Work out the finished part from the listing and answer in its coordinate system (mm). A direction names the side the tool comes from. Give positions to 0.01 mm unless a question says otherwise; leave off trailing zeros. Loops run counter-clockwise (first coordinate to the right, second up) from the corner with the lowest first, then second, coordinate; pieces in that order, holes last. Notation, with made-up numbers: (31.25, 38) - (61.25, 38) arc R24 cw to (61.25, 55) - close; hole circle Ø2 at (-24.75, 44.5). An arc over 180 degrees is marked (long way). One line per item, written item: value.
from build123d import *

# Parameters (mm, degrees)
SKETCH_1_W           = 35.5
SKETCH_1_H           = 24
EXTRUDE_1_DEPTH      = 7
SKETCH_2_W           = 33.2
SKETCH_2_H           = 22.1
CUT_EXTRUDE_1_DEPTH  = 6
CUT_EXTRUDE_2_DEPTH  = 2
EXTRUDE_2_DEPTH      = 6
SKETCH_7_W           = 5
SKETCH_7_H           = 2
EXTRUDE_3_DEPTH      = 5
CUT_EXTRUDE_4_DEPTH  = 2
SKETCH_12_W          = 5.5
SKETCH_12_H          = 2
CUT_EXTRUDE_6_DEPTH  = 6
SKETCH_19_W          = 8
SKETCH_19_H          = 10
USB_DEPTH            = 1.5
SKETCH_25_W          = 0.5
SKETCH_25_H          = 18.1
CUT_EXTRUDE_12_DEPTH = 6
SKETCH_28_W          = 5.5
SKETCH_28_H          = 1.9
CUT_EXTRUDE_13_DEPTH = 6
SKETCH_29_W          = 6
SKETCH_29_H          = 2
CUT_EXTRUDE_14_DEPTH = 5
SKETCH_34_W          = 7
SKETCH_34_H          = 10
EXTRUDE_10_DEPTH     = 3.3
SKETCH_35_W          = 0.5
SKETCH_35_H          = 10
CUT_EXTRUDE_15_DEPTH = 3
SKETCH_37_W          = 4.5
SKETCH_37_H          = 2
EXTRUDE_12_DEPTH     = 5.5
SKETCH_38_W          = 1.5
SKETCH_38_H          = 2.5
CUT_EXTRUDE_16_DEPTH = 2
SKETCH_39_W          = 4.5
SKETCH_39_H          = 1
CUT_EXTRUDE_17_DEPTH = 5.5
SKETCH_40_W          = 4.5
SKETCH_40_H          = 3
EXTRUDE_13_DEPTH     = 1.5
FILLET_2_R           = 1
SKETCH_41_W          = 4.5
SKETCH_41_H          = 2
EXTRUDE_14_DEPTH     = 5.5
SKETCH_42_W          = 1.5
SKETCH_42_H          = 2.5
CUT_EXTRUDE_18_DEPTH = 2
SKETCH_43_W          = 4.5
SKETCH_43_H          = 1
CUT_EXTRUDE_19_DEPTH = 5.5
SKETCH_44_W          = 4.5
SKETCH_44_H          = 3
EXTRUDE_15_DEPTH     = 1.5
FILLET_3_R           = 1
EXTRUDE_16_DEPTH     = 2
SKETCH_50_W          = 5.5
SKETCH_50_H          = 2
CUT_EXTRUDE_20_DEPTH = 2
SKETCH_51_W          = 5.5
SKETCH_51_H          = 2
CUT_EXTRUDE_21_DEPTH = 2
SKETCH_54_W          = 2
SKETCH_54_H          = 0.95
EXTRUDE_19_DEPTH     = 2
SKETCH_55_W          = 2
SKETCH_55_H          = 1
EXTRUDE_20_DEPTH     = 15.5
SKETCH_56_W          = 2
SKETCH_56_H          = 1
EXTRUDE_21_DEPTH     = 2
SKETCH_57_W          = 2
SKETCH_57_H          = 1
EXTRUDE_22_DEPTH     = 7.5
SKETCH_58_W          = 1.5
SKETCH_58_H          = 1.9
SKETCH_58_H_2        = 2
EXTRUDE_24_DEPTH     = 2
SKETCH_59_W          = 6
SKETCH_59_H          = 1
EXTRUDE_25_DEPTH     = 1
CUT_EXTRUDE_22_DEPTH = 0.3
CUT_EXTRUDE_23_DEPTH = 0.3


with BuildPart() as part:
    # Sketch 1 → Extrude 1 (new body)
    with BuildSketch(Plane.XY):
        Rectangle(SKETCH_1_W, SKETCH_1_H)
    extrude(amount=EXTRUDE_1_DEPTH)

    # Sketch 2 → Cut-Extrude 1 (cut)
    with BuildSketch(Plane.XY.offset(7)):
        with Locations((0.25, 0.05)):
            Rectangle(SKETCH_2_W, SKETCH_2_H)
    extrude(amount=-CUT_EXTRUDE_1_DEPTH, mode=Mode.SUBTRACT)

    # Sketch 3 → Cut-Extrude 2 (cut)
    with BuildSketch(Plane.ZY.offset(17.75)):
        with BuildLine():
            Line((6, 7.45), (6, 1.95))
            ThreePointArc((6, 1.95), (4.25, 0.2), (2.5, 1.95))
            Line((2.5, 1.95), (2.5, 7.45))
            ThreePointArc((2.5, 7.45), (4.25, 9.2), (6, 7.45))
        make_face()
    extrude(amount=-CUT_EXTRUDE_2_DEPTH, mode=Mode.SUBTRACT)

    # Sketch 6 → Extrude 2 (add)
    with BuildSketch(Plane.XY.offset(1)):
        Polygon((-16.35, 10.1), (15.85, 10.1), (15.85, -10), (-16.35, -10), (-16.35, -11), (16.85, -11), (16.85, 11.1), (-16.35, 11.1), align=None)
    extrude(amount=EXTRUDE_2_DEPTH)

    # Sketch 7 → Extrude 3 (add)
    with BuildSketch(Plane.XY.offset(1)):
        with Locations((13.35, 9.1)):
            Rectangle(SKETCH_7_W, SKETCH_7_H)
    extrude(amount=EXTRUDE_3_DEPTH)

    # Sketch 10 → Cut-Extrude 4 (cut)
    with BuildSketch(Plane.ZY.offset(-15.85)):
        with BuildLine():
            Line((1.5, -6.45), (1.5, 4.55))
            ThreePointArc((1.5, 4.55), (3.75, 6.8), (6, 4.55))
            Line((6, 4.55), (6, -6.45))
            ThreePointArc((6, -6.45), (3.75, -8.7), (1.5, -6.45))
        make_face()
    extrude(amount=-CUT_EXTRUDE_4_DEPTH, mode=Mode.SUBTRACT)

    # Sketch 12 → Cut-Extrude 6 (cut)
    with BuildSketch(Plane.XY.offset(7)):
        with Locations((-1.6, -11)):
            Rectangle(SKETCH_12_W, SKETCH_12_H)
    extrude(amount=-CUT_EXTRUDE_6_DEPTH, mode=Mode.SUBTRACT)

    # Sketch 19 → USB (add)
    with BuildSketch(Plane.XY.offset(1)):
        with Locations((-12.25, 5.1)):
            Rectangle(SKETCH_19_W, SKETCH_19_H)
    extrude(amount=USB_DEPTH)

    # Sketch 25 → Cut-Extrude 12 (cut)
    with BuildSketch(Plane.XY.offset(7)):
        with Locations((16.1, -0.95)):
            Rectangle(SKETCH_25_W, SKETCH_25_H)
    extrude(amount=-CUT_EXTRUDE_12_DEPTH, mode=Mode.SUBTRACT)

    # Sketch 28 → Cut-Extrude 13 (cut)
    with BuildSketch(Plane.XY.offset(7)):
        with Locations((-5.1, 11.05)):
            Rectangle(SKETCH_28_W, SKETCH_28_H)
    extrude(amount=-CUT_EXTRUDE_13_DEPTH, mode=Mode.SUBTRACT)

    # Sketch 29 → Cut-Extrude 14 (cut)
    with BuildSketch(Plane.XY.offset(7)):
        with Locations((2.65, 11)):
            Rectangle(SKETCH_29_W, SKETCH_29_H)
    extrude(amount=-CUT_EXTRUDE_14_DEPTH, mode=Mode.SUBTRACT)

    # Sketch 34 → Extrude 10 (add)
    with BuildSketch(Plane.XY.offset(1)):
        with Locations((-12.75, -5)):
            Rectangle(SKETCH_34_W, SKETCH_34_H)
    extrude(amount=EXTRUDE_10_DEPTH)

    # Sketch 35 → Cut-Extrude 15 (cut)
    with BuildSketch(Plane.XY.offset(7)):
        with Locations((-16.5, 5.1)):
            Rectangle(SKETCH_35_W, SKETCH_35_H)
    extrude(amount=-CUT_EXTRUDE_15_DEPTH, mode=Mode.SUBTRACT)

    # Sketch 37 → Extrude 12 (add)
    with BuildSketch(Plane.XY.offset(1)):
        with Locations((-1.6, -11)):
            Rectangle(SKETCH_37_W, SKETCH_37_H)
    extrude(amount=EXTRUDE_12_DEPTH)

    # Sketch 38 → Cut-Extrude 16 (cut)
    with BuildSketch(Plane.XZ.offset(12)):
        with Locations((-3.1, 2.25)):
            Rectangle(SKETCH_38_W, SKETCH_38_H)
        with Locations((-0.1, 2.25)):
            Rectangle(SKETCH_38_W, SKETCH_38_H)
    extrude(amount=-CUT_EXTRUDE_16_DEPTH, mode=Mode.SUBTRACT)

    # Sketch 39 → Cut-Extrude 17 (cut)
    with BuildSketch(Plane.XY.offset(6.5)):
        with Locations((-1.6, -10.5)):
            Rectangle(SKETCH_39_W, SKETCH_39_H)
    extrude(amount=-CUT_EXTRUDE_17_DEPTH, mode=Mode.SUBTRACT)

    # Sketch 40 → Extrude 13 (add)
    with BuildSketch(Plane.XZ.offset(12)):
        with Locations((-1.6, 5)):
            Rectangle(SKETCH_40_W, SKETCH_40_H)
    extrude(amount=EXTRUDE_13_DEPTH)

    # Fillet 2
    fillet_2_edges = [part.edges().sort_by_distance(p)[0] for p in [
        (-3.85, -13.5, 5),
        (-1.6, -13.5, 3.5),
        (0.65, -13.5, 5),
        (-1.6, -13.5, 6.5),
    ]]
    fillet(fillet_2_edges, radius=FILLET_2_R)

    # Sketch 41 → Extrude 14 (add)
    with BuildSketch(Plane.XY.offset(1)):
        with Locations((-5.1, 11)):
            Rectangle(SKETCH_41_W, SKETCH_41_H)
    extrude(amount=EXTRUDE_14_DEPTH)

    # Sketch 42 → Cut-Extrude 18 (cut)
    with BuildSketch(Plane(origin=(0, 12, 0), x_dir=(1, 0, 0), z_dir=(0, 1, 0))):
        with Locations((-6.6, -2.25)):
            Rectangle(SKETCH_42_W, SKETCH_42_H)
        with Locations((-3.6, -2.25)):
            Rectangle(SKETCH_42_W, SKETCH_42_H)
    extrude(amount=-CUT_EXTRUDE_18_DEPTH, mode=Mode.SUBTRACT)

    # Sketch 43 → Cut-Extrude 19 (cut)
    with BuildSketch(Plane.XY.offset(6.5)):
        with Locations((-5.1, 10.5)):
            Rectangle(SKETCH_43_W, SKETCH_43_H)
    extrude(amount=-CUT_EXTRUDE_19_DEPTH, mode=Mode.SUBTRACT)

    # Sketch 44 → Extrude 15 (add)
    with BuildSketch(Plane(origin=(0, 12, 0), x_dir=(1, 0, 0), z_dir=(0, 1, 0))):
        with Locations((-5.1, -5)):
            Rectangle(SKETCH_44_W, SKETCH_44_H)
    extrude(amount=EXTRUDE_15_DEPTH)

    # Fillet 3
    fillet_3_edges = [part.edges().sort_by_distance(p)[0] for p in [
        (-7.35, 13.5, 5),
        (-5.1, 13.5, 6.5),
        (-2.85, 13.5, 5),
        (-5.1, 13.5, 3.5),
    ]]
    fillet(fillet_3_edges, radius=FILLET_3_R)

    # Sketch 45 → Extrude 16 (add)
    with BuildSketch(Plane.XY.offset(7)):
        Polygon((-7.85, 10.1), (-16.35, 10.1), (-16.35, 11.1), (-7.85, 11.05), (-2.25, 11.05), (-0.35, 11.05), (-0.35, 10.1), (-2.35, 10.1), align=None)
        Polygon((1.25, -11), (-16.35, -11), (-16.35, -10), (1.15, -10), (15.85, -10), (15.85, 10.1), (5.65, 10.1), (5.65, 11), (16.65, 11), (16.65, 10), (16.65, -11), align=None)
    extrude(amount=EXTRUDE_16_DEPTH)

    # Sketch 46 → Revolve 1 (revolve)
    with BuildSketch(Plane.XZ.offset(11)):
        with BuildLine():
            Line((-11.25, 8), (-10.25, 8))
            ThreePointArc((-10.25, 8), (-10.75, 8.5), (-11.25, 8))
        make_face()
    revolve(axis=Axis((-11.25, -11, 8), (1, 0, 0)))

    # Sketch 47 → Revolve 2 (revolve)
    with BuildSketch(Plane.XZ.offset(11)):
        with BuildLine():
            Line((11.25, 8), (10.25, 8))
            ThreePointArc((10.25, 8), (10.75, 8.5), (11.25, 8))
        make_face()
    revolve(axis=Axis((11.25, -11, 8), (-1, 0, 0)))

    # Sketch 48 → Revolve 3 (revolve)
    with BuildSketch(Plane(origin=(0, 11.05, 0), x_dir=(1, 0, 0), z_dir=(0, 1, 0))):
        with BuildLine():
            Line((-11.25, -8), (-10.25, -8))
            ThreePointArc((-10.25, -8), (-10.75, -7.5), (-11.25, -8))
        make_face()
    revolve(axis=Axis((-11.25, 11.05, 8), (1, 0, 0)))

    # Sketch 49 → Revolve 4 (revolve)
    with BuildSketch(Plane(origin=(0, 11, 0), x_dir=(1, 0, 0), z_dir=(0, 1, 0))):
        with BuildLine():
            Line((10.25, -8), (11.25, -8))
            ThreePointArc((11.25, -8), (10.75, -7.5), (10.25, -8))
        make_face()
    revolve(axis=Axis((10.25, 11, 8), (1, 0, 0)))

    # Sketch 50 → Cut-Extrude 20 (cut)
    with BuildSketch(Plane.XZ.offset(-10.1)):
        with Locations((-5.1, 8)):
            Rectangle(SKETCH_50_W, SKETCH_50_H)
    extrude(amount=-CUT_EXTRUDE_20_DEPTH, mode=Mode.SUBTRACT)

    # Sketch 51 → Cut-Extrude 21 (cut)
    with BuildSketch(Plane.XZ.offset(11)):
        with Locations((-1.6, 8)):
            Rectangle(SKETCH_51_W, SKETCH_51_H)
    extrude(amount=-CUT_EXTRUDE_21_DEPTH, mode=Mode.SUBTRACT)

    # Sketch 54 → Extrude 19 (add)
    with BuildSketch(Plane.XY.offset(7)):
        with Locations((-8.85, 11.525)):
            Rectangle(SKETCH_54_W, SKETCH_54_H)
    extrude(amount=EXTRUDE_19_DEPTH)

    # Sketch 55 → Extrude 20 (add)
    with BuildSketch(Plane(origin=(-7.85, 0, 0), x_dir=(0, 0, -1), z_dir=(1, 0, 0))):
        with Locations((-8, 11.5)):
            Rectangle(SKETCH_55_W, SKETCH_55_H)
    extrude(amount=EXTRUDE_20_DEPTH)

    # Sketch 56 → Extrude 21 (add)
    with BuildSketch(Plane.XY.offset(7)):
        with Locations((-5.35, -11.5)):
            Rectangle(SKETCH_56_W, SKETCH_56_H)
    extrude(amount=EXTRUDE_21_DEPTH)

    # Sketch 57 → Extrude 22 (add)
    with BuildSketch(Plane(origin=(-4.35, 0, 0), x_dir=(0, 0, -1), z_dir=(1, 0, 0))):
        with Locations((-8, -11.5)):
            Rectangle(SKETCH_57_W, SKETCH_57_H)
    extrude(amount=EXTRUDE_22_DEPTH)

    # Sketch 58 → Extrude 24 (add)
    with BuildSketch(Plane.XY.offset(1)):
        with Locations((-7.1, 11.05)):
            Rectangle(SKETCH_58_W, SKETCH_58_H)
        with Locations((-3.1, 11.05)):
            Rectangle(SKETCH_58_W, SKETCH_58_H)
        with Locations((-3.6, -11)):
            Rectangle(SKETCH_58_W, SKETCH_58_H_2)
        with Locations((0.4, -11)):
            Rectangle(SKETCH_58_W, SKETCH_58_H_2)
    extrude(amount=EXTRUDE_24_DEPTH)

    # Sketch 59 → Extrude 25 (add)
    with BuildSketch(Plane(origin=(0, 0, 7), x_dir=(-1, 0, 0), z_dir=(0, 0, -1))):
        with Locations((-2.65, 11.5)):
            Rectangle(SKETCH_59_W, SKETCH_59_H)
    extrude(amount=EXTRUDE_25_DEPTH)

    # Sketch 61 → Cut-Extrude 22 (cut)
    with BuildSketch(Plane(origin=(0, 12, 0), x_dir=(1, 0, 0), z_dir=(0, 1, 0))):
        with BuildLine():
            Line((-9.6, -6.159611152), (-9.6, -4.5))
            ThreePointArc((-9.6, -4.5), (-9.85, -4.25), (-10.1, -4.5))
            Line((-10.1, -4.5), (-10.1, -6.159611152))
            ThreePointArc((-10.1, -6.159611152), (-9.85, -6.409611152), (-9.6, -6.159611152))
        make_face()
        with BuildLine():
            ThreePointArc((-9.101668523, -5.8), (-9.85, -3), (-10.598331477, -5.8))
            ThreePointArc((-10.598331477, -5.8), (-10.274165739, -5.624165739), (-10.45, -5.3))
            ThreePointArc((-10.45, -5.3), (-9.85, -3.5), (-9.25, -5.3))
            ThreePointArc((-9.25, -5.3), (-9.425834261, -5.624165739), (-9.101668523, -5.8))
        make_face()
    extrude(amount=-CUT_EXTRUDE_22_DEPTH, mode=Mode.SUBTRACT)

    # Sketch 60 → Cut-Extrude 23 (cut)
    with BuildSketch(Plane(origin=(0, 12, 0), x_dir=(1, 0, 0), z_dir=(0, 1, 0))):
        Polygon((4.45, -8.8), (4.45, -7.2), (5.049338639, -7.8), (5.403086939, -7.446641626), (4.200665644, -6.242893478), (2.995979535, -7.4462517), (3.349337909, -7.8), (3.95, -7.2), (3.95, -8.8), align=None)
        Polygon((1.35, -6.242893478), (0.85, -6.242893478), (0.85, -7.842893478), (0.250661361, -7.242893478), (-0.103086939, -7.596251853), (1.099334356, -8.8), (2.304020465, -7.596641778), (1.950662091, -7.242893478), (1.35, -7.842893478), align=None)
    extrude(amount=-CUT_EXTRUDE_23_DEPTH, mode=Mode.SUBTRACT)


solid = part.part
1. For faces 1 (the cylindrical face through (-17.22, 0.29, 3.69)), 2 (the flat face through (-4.35, -11, 5)), 3 (the flat face through (-2, -11, 8)), determine the directions among +Z, -Z, +X, -X, +Y, -Y from which every point of the face is accessible in a straight line to the end or side of a thin tool.
Output:
face 1: +X, -X
face 2: none
face 3: +Z
2. Section D-D (z = 0.5) is taken. Write down the section's boundary in (x, y), and give its area (3 significant figures).
Output:
outline: (-17.75, -12) - (17.75, -12) - (17.75, 12) - (-17.75, 12) - close
area: 852 mm²
3. Section B-B (x = 9.5) is taken. Write down the section's boundary in (y, z), and give its area (3 significant figures).
Output:
outline: (-12, 0) - (12, 0) - (12, 7) - (11, 7) - (11, 9) - (10.1, 9) - (10.1, 1) - (-10, 1) - (-10, 9) - (-11, 9) - (-11, 7) - (-12, 7) - close
area: 51.2 mm²
4. Flat-ended cylindrical pins translate along their axes: pin 1 Ø1.5 at (x, y) = (4.5, -0.5) entering from +Z; pin 2 Ø2 at (x, z) = (-2, 7.5) entering from +Y; pin 3 Ø1 at (y, z) = (-2.5, 8) entering from +X. Find the tip coordinate at first contact, or state that the pin passes through.
Output:
pin 1: stops at z = 1
pin 2: stops at y = 12
pin 3: stops at x = 16.65
5. Section A-A (y = 2.5) is taken. Write down the section's boundary in (x, z).
Output:
outline: (-17.75, 0) - (17.75, 0) - (17.75, 1.5) - (16.35, 1.5) - (16.35, 1) - (-8.25, 1) - (-8.25, 2.5) - (-16.25, 2.5) - (-16.25, 1) - (-16.35, 1) - (-16.35, 2.5) - (-17.75, 2.5) - close; (-17.75, 6) - (-16.75, 6) - (-16.75, 7) - (-17.75, 7) - close; (15.85, 7) - (16.35, 7) - (16.35, 6) - (17.75, 6) - (17.75, 7) - (16.65, 7) - (16.65, 9) - (15.85, 9) - close
6. Section C-C (y = -9.25) is taken. Write down the section's boundary in (x, z), and give its area (3 significant figures).
Output:
outline: (-17.75, 0) - (17.75, 0) - (17.75, 7) - (16.65, 7) - (16.65, 9) - (15.85, 9) - (15.85, 7) - (16.35, 7) - (16.35, 1) - (-9.25, 1) - (-9.25, 4.3) - (-16.25, 4.3) - (-16.25, 1) - (-16.35, 1) - (-16.35, 7) - (-17.75, 7) - close
area: 77.0 mm²
7. The mould has two halves that part along Y. Classify faces 4 (the flat face through (0, 0, 0)), 5 (the cylindrical face through (-5.068, 13.199, 6.215)), 6 (the flat face through (-17, 5, 6)), 7 (the flat face through (1.15, -11, 5)): released by +Y, released by -Y, zero draft, split by the parting line, or undercut.
Output:
face 4: zero draft
face 5: released by +Y
face 6: undercut
face 7: undercut
8. Find the intervals of material crossed by line 1 along Y through (x, z) = (6.5, 1.5); line 2 along Y through (x, z) = (2, 7.75); line 3 along X through (y, z) = (-5.25, 6.75), in increasing order.
Output:
line 1: y = -12 to -10, 10.1 to 12
line 2: y = -12 to -10, 11 to 11.7
line 3: x = -17.75 to -16.35, 16.35 to 17.75
